Here's how the part is built. I have some questions about the finished solid (model axes, mm). A direction names the side the tool comes from. Round coordinates to 2 decimals unless told otherwise and drop trailing zeros. Loops run counter-clockwise (first coordinate to the right, second up) from the corner with the lowest first, then second, coordinate; pieces in that order, holes last. Notation, with made-up numbers: M -39,-27 L -28,-27 A19 ccw -28,1 Z; hole C -8,28.5 d4. An arc over 180 degrees is marked long. Use a Markdown table: item, result.
```python
from build123d import *

# Parameters (mm, degrees)
SKETCH_R     = 2.75
PAD_DEPTH    = 3
SKETCH001_R  = 1.5
PAD001_DEPTH = 25
POCKET_DEPTH = 4


with BuildPart() as part:
    # Sketch → Pad (new body)
    with BuildSketch(Plane.XY):
        Circle(SKETCH_R)
    extrude(amount=PAD_DEPTH)

    # Sketch001 (on Face2 of Pad) → Pad001 (join)
    with BuildSketch(Plane(origin=(0, 0, 0), x_dir=(1, 0, 0), z_dir=(0, 0, -1))):
        Circle(SKETCH001_R)
    extrude(amount=PAD001_DEPTH)

    # Sketch002 (on DatumPlane) → Pocket (cut)
    with BuildSketch(Plane.XY.offset(3)):
        Polygon((0.721688, -1.25), (1.443376, 0), (0.721688, 1.25), (-0.721688, 1.25), (-1.443376, 0), (-0.721688, -1.25), align=None)
    extrude(amount=-POCKET_DEPTH, mode=Mode.SUBTRACT)


solid = part.part
```
Q1. Imagine slicing it at A-A, the plane x = 0. Please give me the cut outline in (y, z), then the cut area to 3 significant figures.
Return value:
| item | result |
|---|---|
| outline | M -2.75,0 L -1.5,0 L -1.5,-25 L 1.5,-25 L 1.5,0 L 2.75,0 L 2.75,3 L 1.25,3 L 1.25,-1 L -1.25,-1 L -1.25,3 L -2.75,3 Z |
| area | 81.5 mm^2 |
Q2. Will these pins go through, and if not, where does the flat tip stop? P1, Ø1, axis at x = 0, z = -13, coming from the -Y side; P2, Ø1, axis at y = -1, z = -5.5, coming from the +X side.
Return value:
| item | result |
|---|---|
| P1 | stops at y = -1.5 |
| P2 | stops at x = 1.41 |
Q3. Imagine slicing it at D-D, the plane y = -2.1. Please give me the cut outline in (x, z), then the cut area to 3 significant figures.
Return value:
| item | result |
|---|---|
| outline | M -1.78,0 L 1.78,0 L 1.78,3 L -1.78,3 Z |
| area | 10.7 mm^2 |
Q4. I need wall thicknesses on line 1 (X direction, y = 0, z = -22); line 2 (Z direction, x = 1.8, y = 0.6); line 3 (Z direction, x = 0.65, y = 1.05). Which ranges of each line are inside material? Lowest first, please. Write a range as from..to.
Return value:
| item | result |
|---|---|
| line 1 | x = -1.5..1.5 |
| line 2 | z = 0..3 |
| line 3 | z = -25..-1 |
Q5. Imagine slicing it at B-B, the plane y = -0.8. Please give me the cut outline in (x, z).
Return value:
| item | result |
|---|---|
| outline | M -2.63,0 L -1.27,0 L -1.27,-25 L 1.27,-25 L 1.27,0 L 2.63,0 L 2.63,3 L 0.98,3 L 0.98,-1 L -0.98,-1 L -0.98,3 L -2.63,3 Z |
Q6. We'd pull the mould along Y, two halves only. Please class faces 4 (the flat face through (-1.088, -0.616, 1.028)), 5 (the cylindrical face through (-1.5, -0.07, -12.32)), 6 (the flat face through (-1.3, -0.6, 3)): pulls with the +Y half, pulls with the -Y half, needs draft (parallel to the pull), parting line crosses it, or undercut.
Return value:
| item | result |
|---|---|
| face 4 | undercut |
| face 5 | parting line crosses it |
| face 6 | needs draft |
Q7. Imagine slicing it at C-C, the plane z = -4.5. Please give me the cut outline in (x, y).
Return value:
| item | result |
|---|---|
| outline | C 0,0 d3 |
Q8. For faces 1 (the flat face through (1.2, -1.2, 0)), 2 (the flat face through (0, 0, -25)), 3 (the flat face through (-1.08, 0.63, 1.03)), which set-ups out of +Z, -Z, +X, -X, +Y, -Y let a thin tool reach every point of the face, with its end or its side?
Return value:
| item | result |
|---|---|
| face 1 | -Z |
| face 2 | -Z, +X, -X, +Y, -Y |
| face 3 | +Z |
